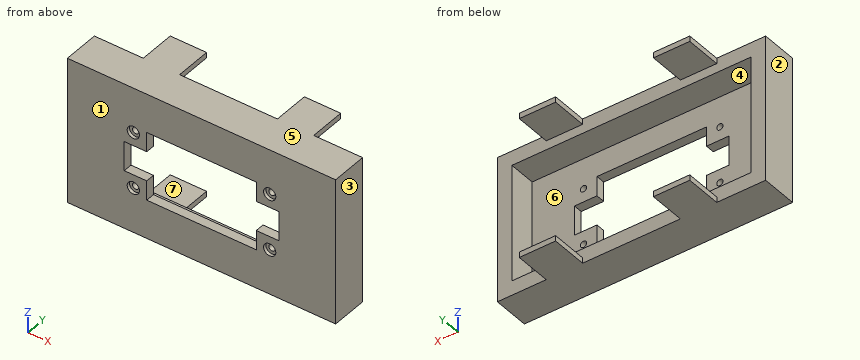
```python
from build123d import *

# Parameters (mm, degrees)
SKETCH1_W                                           = 147.57
SKETCH1_H                                           = 80.42
BOSS_EXTRUDE1_DEPTH                                 = 20
SKETCH2_W                                           = 131.57
SKETCH2_H                                           = 64.42
CUT_EXTRUDE1_DEPTH                                  = 15
CBORE_FOR_4_BINDING_HEAD_MACHINE_SCREW1_D           = 3.4544
CBORE_FOR_4_BINDING_HEAD_MACHINE_SCREW1_CBORE_D     = 6.74624
CBORE_FOR_4_BINDING_HEAD_MACHINE_SCREW1_CBORE_DEPTH = 1.7272
CUT_EXTRUDE2_DEPTH                                  = 170.246215024
SKETCH6_W                                           = 20
SKETCH6_H                                           = 3
BOSS_EXTRUDE2_DEPTH                                 = 20
MIRROR2_COPY_1_SKETCH_W                             = 20
MIRROR2_COPY_1_SKETCH_H                             = 3
MIRROR2_COPY_1_DEPTH                                = 20


with BuildPart() as part:
    # Sketch1 → Boss-Extrude1 (new body)
    with BuildSketch(Plane(origin=(0, 0, 0), x_dir=(1, 0, 0), z_dir=(0, 1, 0))):
        with Locations((73.785, 40.21)):
            Rectangle(SKETCH1_W, SKETCH1_H)
    extrude(amount=BOSS_EXTRUDE1_DEPTH)

    # Sketch2 → Cut-Extrude1 (cut)
    with BuildSketch(Plane(origin=(0, 20, 0), x_dir=(1, 0, 0), z_dir=(0, 1, 0))):
        with Locations((73.785, 40.21)):
            Rectangle(SKETCH2_W, SKETCH2_H)
    extrude(amount=-CUT_EXTRUDE1_DEPTH, mode=Mode.SUBTRACT)

    # CBORE for #4 Binding Head Machine Screw1 (through all)
    with Locations(Plane(origin=(36.285, 0, -24.71), x_dir=(0, 0, -1), z_dir=(0, -1, 0))):
        with Locations((0, 0), (31, 0), (0, 75), (31, 75)):
            CounterBoreHole(CBORE_FOR_4_BINDING_HEAD_MACHINE_SCREW1_D / 2, CBORE_FOR_4_BINDING_HEAD_MACHINE_SCREW1_CBORE_D / 2, CBORE_FOR_4_BINDING_HEAD_MACHINE_SCREW1_CBORE_DEPTH)

    # Sketch5 → Cut-Extrude2 (cut, through all)
    with BuildSketch(Plane.XZ):
        Polygon((103.91188, -32.08312), (103.91188, -21.33688), (43.65812, -21.33688), (43.65812, -32.08312), (31.285, -32.08312), (31.285, -48.33688), (43.65812, -48.33688), (43.65812, -59.08312), (103.91188, -59.08312), (103.91188, -48.33688), (116.285, -48.33688), (116.285, -32.08312), align=None)
    extrude(amount=-CUT_EXTRUDE2_DEPTH, mode=Mode.SUBTRACT)

    # Sketch6 → Boss-Extrude2 (add)
    with BuildSketch(Plane(origin=(0, 20, 0), x_dir=(1, 0, 0), z_dir=(0, 1, 0))):
        with Locations((36.8925, 78.92)):
            Rectangle(SKETCH6_W, SKETCH6_H)
    boss_extrude2 = extrude(amount=BOSS_EXTRUDE2_DEPTH)

    # Mirror1: Boss-Extrude2 across plane
    add(boss_extrude2.mirror(Plane(origin=(73.785, 0, 0), x_dir=(0, 0, 1), z_dir=(1, 0, 0))))

    # Mirror2: Boss-Extrude2 across plane
    add(boss_extrude2.mirror(Plane(origin=(0, 0, -40.21), x_dir=(1, 0, 0), z_dir=(0, 0, -1))))

    # Mirror2 copy 1 sketch → Mirror2 copy 1 (add)
    with BuildSketch(Plane(origin=(147.57, 20, -80.42), x_dir=(-1, 0, 0), z_dir=(0, 1, 0))):
        with Locations((36.8925, 78.92)):
            Rectangle(MIRROR2_COPY_1_SKETCH_W, MIRROR2_COPY_1_SKETCH_H)
    extrude(amount=MIRROR2_COPY_1_DEPTH)


solid = part.part
```
Geometry: final body of the model. Coordinates: model frame, mm. Face numbers are marked on the shaded views. A direction names the side the tool comes from. Coordinates: 2 decimals unless noted, no trailing zeros. Order: outer loops, then holes, each group sorted by start corner. A loop starts at its lowest first (then second) coordinate and runs counter-clockwise, first axis right, second up. Notation, with made-up numbers: M -34.5,86.5 L -3.5,86.5 A16 ccw -3.5,114.5 Z; hole C -15,62.5 d1. An arc over 180 degrees is marked long. Answer in a Markdown table with one row per item. Add a question column.
Q1. Line query: L1, parallel to X at y = 0.85, z = -24.71; L2, parallel to Z at x = 123.5, y = 17.5; L3, parallel to X at y = 17, z = -70. Output: solid intervals per line, ascending.
Q2. Section query B-B on x = 90. Return the cut outline in (y, z), and give its area (3 significant figures).
Q3. Contact query for flat-ended pins moving along their axis: P1, Ø3.5, axis at y = 28.5, z = -1, coming from the +X side; P2, Ø8, axis at x = 36.285, z = -55.71, coming from the +Y side; P3, Ø2, axis at x = 35, z = -55, coming from the -Y side; P4, Ø1.5, axis at x = 37.5, y = 2, coming from the +Z side. Output: stop coordinate, or through.
Q4. Section query D-D on z = -68.5. Return the cut outline in (x, y).
Q5. Mould query, pull axis X, two halves, no side actions, for the marked faces 1, 2, 3 and 4. Classes: released by +X, released by -X, zero draft, split by the parting line, or undercut.
Q6. Section query A-A on y = 36.5. Return the cut outline in (x, z), and give its area (3 significant figures).
Q7. Section query C-C on z = -24.71. Return the cut outline in (x, y).
Q8. Reachability of the marked faces 5, 6 and 7 from +Z, -Z, +X, -X, +Y, -Y: full face, straight path, thin tool, end or side. Return the list, or none.
Completed:
| question | item | result |
|---|---|---|
| 1 | L1 | x = 0 to 32.91, 39.66 to 43.66, 103.91 to 107.91, 114.66 to 147.57 |
| 1 | L2 | z = -80.42 to -72.42, -8 to 0 |
| 1 | L3 | x = 0 to 8, 139.57 to 147.57 |
| 2 | outline | M 0,-80.42 L 20,-80.42 L 20,-72.42 L 5,-72.42 L 5,-59.08 L 0,-59.08 Z; M 0,-21.34 L 5,-21.34 L 5,-8 L 20,-8 L 20,0 L 0,0 Z |
| 2 | area | 453 mm2 |
| 3 | P1 | stops at x = 120.68 |
| 3 | P2 | stops at y = 5 |
| 3 | P3 | stops at y = 1.73 |
| 3 | P4 | stops at z = 0 |
| 4 | outline | M 0,0 L 147.57,0 L 147.57,20 L 139.57,20 L 139.57,5 L 8,5 L 8,20 L 0,20 Z |
| 5 | face 1 | zero draft |
| 5 | face 2 | released by -X |
| 5 | face 3 | released by +X |
| 5 | face 4 | undercut |
| 6 | outline | M 26.89,-80.42 L 46.89,-80.42 L 46.89,-77.42 L 26.89,-77.42 Z; M 26.89,-3 L 46.89,-3 L 46.89,0 L 26.89,0 Z; M 100.68,-80.42 L 120.68,-80.42 L 120.68,-77.42 L 100.68,-77.42 Z; M 100.68,-3 L 120.68,-3 L 120.68,0 L 100.68,0 Z |
| 6 | area | 240 mm2 |
| 7 | outline | M 0,0 L 32.91,0 L 32.91,1.73 L 34.56,1.73 L 34.56,5 L 8,5 L 8,20 L 0,20 Z; M 38.01,1.73 L 39.66,1.73 L 39.66,0 L 43.66,0 L 43.66,5 L 38.01,5 Z; M 103.91,0 L 107.91,0 L 107.91,1.73 L 109.56,1.73 L 109.56,5 L 103.91,5 Z; M 113.01,1.73 L 114.66,1.73 L 114.66,0 L 147.57,0 L 147.57,20 L 139.57,20 L 139.57,5 L 113.01,5 Z |
| 8 | face 5 | +Z, +X, -X, +Y, -Y |
| 8 | face 6 | +Y |
| 8 | face 7 | +X, -X, +Y |
